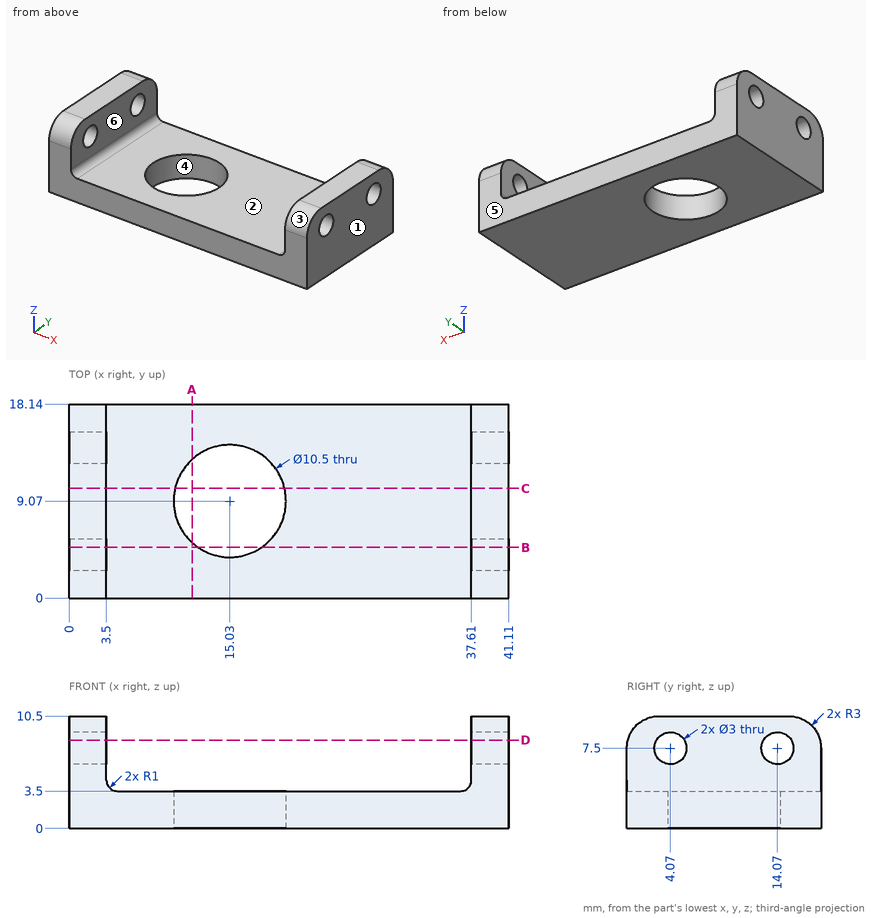
Check sheet for the drawn part. Datum: minimum x, y, z corner. Units: mm. A direction names the side the tool comes from. Round coordinates to 2 decimals unless told otherwise and drop trailing zeros. Loops run counter-clockwise (first coordinate to the right, second up) from the corner with the lowest first, then second, coordinate; pieces in that order, holes last. Notation, with made-up numbers: (72, -12) - (130, -12) arc R31 ccw to (130, 16) - close; hole circle Ø4 at (44.5, 71). An arc over 180 degrees is marked (long way). Write each question's results on one line, items separated by ' | '. Start each with the question number.
Q1. Cross-section at A-A on x = 11.5. Enter the section's corners in (y, z), and give its area (3 significant figures).
Q2. Cross-section at D-D on z = 8.25. Enter the section's corners in (x, y), and give its area (3 significant figures).
Q3. Access from +Z, -Z, +X, -X, +Y, -Y to the whole of each face (thin tool, end or side, straight path). Record for the marked faces 1 and 2.
Q4. Thickness scan on line 1 (Y direction, x = 38.4, z = 7.5); line 2 (Z direction, x = 40.3, y = 14.07); line 3 (Y direction, x = 15.03, z = 2). Record the ranges inside material, lowest first. Write a range as [from, to].
Q5. Gauge pin test, flat end, axial feed: P1, Ø5, axis at y = 14.07, z = 7.5, coming from the -X side. Record the tip position at first contact, or that the pin passes through.
Q6. Cross-section at C-C on y = 10.25. Enter the section's corners in (x, z).
Q7. Cross-section at B-B on y = 4.75. Enter the section's corners in (x, z), and give its area (3 significant figures).
Q8. Release check for a two-part mould opening along Y. For the marked faces 3, 4, 5 and 6 record: +Y half, -Y half, draft (parallel to the pull), parting line (faces both ways), or undercut.
Answers below:
1) outline: (0, 0) - (5.18, 0) - (5.18, 3.5) - (0, 3.5) - close; (12.96, 0) - (18.14, 0) - (18.14, 3.5) - (12.96, 3.5) - close | area: 36.3 mm²
2) outline: (0, 0.1) - (3.5, 0.1) - (3.5, 2.77) - (0, 2.77) - close; (0, 5.37) - (3.5, 5.37) - (3.5, 12.77) - (0, 12.77) - close; (0, 15.37) - (3.5, 15.37) - (3.5, 18.04) - (0, 18.04) - close; (37.61, 0.1) - (41.11, 0.1) - (41.11, 2.77) - (37.61, 2.77) - close; (37.61, 5.37) - (41.11, 5.37) - (41.11, 12.77) - (37.61, 12.77) - close; (37.61, 15.37) - (41.11, 15.37) - (41.11, 18.04) - (37.61, 18.04) - close | area: 89.3 mm²
3) face 1: +Z, -Z, +X, +Y, -Y | face 2: +Z, +Y, -Y
4) line 1: y = [0, 2.57], [5.57, 12.57], [15.57, 18.14] | line 2: z = [0, 6], [9, 10.5] | line 3: y = [0, 3.82], [14.32, 18.14]
5) P1: stops at x = 0
6) outline: (0, 0) - (9.91, 0) - (9.91, 3.5) - (4.5, 3.5) arc R1 cw to (3.5, 4.5) - (3.5, 10.5) - (0, 10.5) - close; (20.15, 0) - (41.11, 0) - (41.11, 10.5) - (37.61, 10.5) - (37.61, 4.5) arc R1 cw to (36.61, 3.5) - (20.15, 3.5) - close
7) outline: (0, 0) - (12.05, 0) - (12.05, 3.5) - (4.5, 3.5) arc R1 cw to (3.5, 4.5) - (3.5, 6.16) - (0, 6.16) - close; (0, 8.84) - (3.5, 8.84) - (3.5, 10.5) - (0, 10.5) - close; (18.01, 0) - (41.11, 0) - (41.11, 6.16) - (37.61, 6.16) - (37.61, 4.5) arc R1 cw to (36.61, 3.5) - (18.01, 3.5) - close; (37.61, 8.84) - (41.11, 8.84) - (41.11, 10.5) - (37.61, 10.5) - close | area: 154 mm²
8) face 3: -Y half | face 4: undercut | face 5: +Y half | face 6: draft
